Could you check a few things on this drawing? It's one solid part, dimensions in mm from its lowest x, y, z. Give positions to 0.01 mm unless a question says otherwise; leave off trailing zeros. Order: outer loops, then holes, each group sorted by start corner. A loop starts at its lowest first (then second) coordinate and runs counter-clockwise, first axis right, second up. Notation, with made-up numbers: (26, 18) - (42, 18) arc R30 ccw to (42, 47) - close; hole circle Ø2 at (-18.5, 46). An arc over 180 degrees is marked (long way). One line per question, with ' | ' between items. Start each with the question number.
1. I need wall thicknesses on probe 1 along Z at (x, y) = (19.05, 1.6); probe 2 along Z at (x, y) = (3.5, 3); probe 3 along X at (y, z) = (8.75, 10) (1 decimal). Which ranges of each line are inside material? Lowest first, please. Write a range as from..to.
2. Imagine slicing it at B-B (y = 1.75). Give the number of separate pieces and of enclosed holes in the cut face, and give its area (3 significant figures).
3. Imagine slicing it at C-C (z = 5). Please give me the cut outline in (x, y) (1 decimal), and give its area (3 significant figures).
4. Imagine slicing it at A-A (x = 5.08). Please give me the cut outline in (y, z), and give its area (3 significant figures).
5. For P1, Ø3.5, axis at x = 5.08, z = 10.16, coming from the +Y side; P2, Ø9, axis at x = 19.05, z = 60, coming from the +Y side (1 decimal), each with a flat end and sliding along its axis, tell me the tip position at first contact or that it passes through.
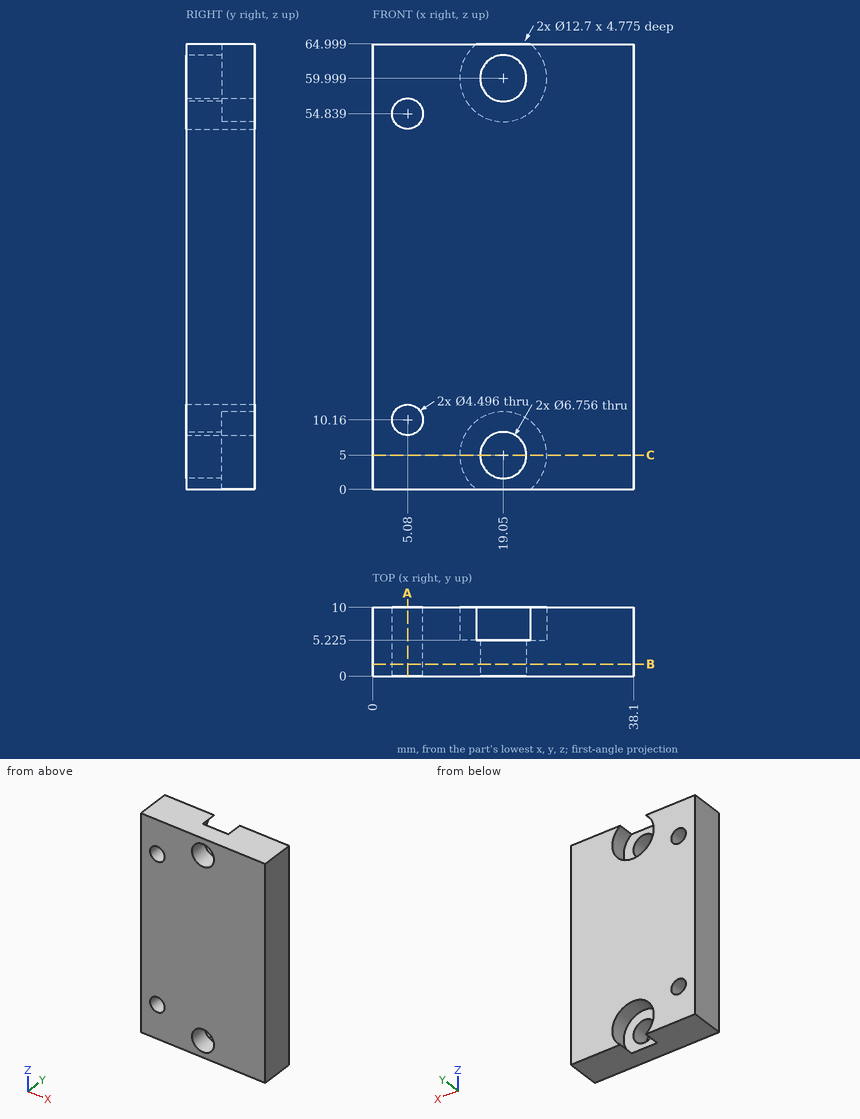
Results found:
1) probe 1: z = 0..1.62, 8.38..56.62, 63.38..65 | probe 2: z = 0..8.56, 11.76..53.24, 56.44..65 | probe 3: x = 0..2.8, 7.3..15.1, 23..38.1
2) separate pieces: 1 | enclosed holes: 4 | area: 2,370 mm2
3) outline: (0, 0) - (15.7, 0) - (15.7, 5.2) - (12.7, 5.2) - (12.7, 10) - (0, 10) - close; (22.4, 0) - (38.1, 0) - (38.1, 10) - (25.4, 10) - (25.4, 5.2) - (22.4, 5.2) - close | area: 285 mm2
4) outline: (0, 0) - (10, 0) - (10, 7.91) - (0, 7.91) - close; (0, 12.41) - (10, 12.41) - (10, 52.59) - (0, 52.59) - close; (0, 57.09) - (10, 57.09) - (10, 65) - (0, 65) - close | area: 560 mm2
5) P1: passes through | P2: stops at y = 5.2
